```python
from build123d import *

# Parameters (mm, degrees)
SKETCH1_W           = 30.5
SKETCH1_H           = 10
BOSS_EXTRUDE1_DEPTH = 2.5
SKETCH2_W           = 35.5
SKETCH2_H           = 15
BOSS_EXTRUDE3_DEPTH = 43
SKETCH3_W           = 7
SKETCH3_H           = 3.4
CUT_EXTRUDE1_DEPTH  = 29
SKETCH4_W           = 35.5
SKETCH4_H           = 2.5
BOSS_EXTRUDE4_DEPTH = 10
SKETCH5_W           = 35.5
SKETCH5_H           = 53
SKETCH5_W_2         = 33.5
SKETCH5_H_2         = 51
BOSS_EXTRUDE5_DEPTH = 7
SKETCH6_W           = 10.5
SKETCH6_H           = 45
BOSS_EXTRUDE6_DEPTH = 7
SKETCH7_W           = 5
SKETCH7_H           = 1
SKETCH7_W_2         = 1
SKETCH7_H_2         = 2
CUT_EXTRUDE2_DEPTH  = 7
SKETCH8_W           = 1.6
SKETCH8_H           = 44
CUT_EXTRUDE3_DEPTH  = 2.5


with BuildPart() as part:
    # Sketch1 → Boss-Extrude1 (new body)
    with BuildSketch(Plane(origin=(0, 0, 0), x_dir=(1, 0, 0), z_dir=(0, 1, 0))):
        Rectangle(SKETCH1_W, SKETCH1_H)
    extrude(amount=BOSS_EXTRUDE1_DEPTH)

    # Sketch2 → Boss-Extrude3 (add)
    with BuildSketch(Plane(origin=(0, 0, 0), x_dir=(1, 0, 0), z_dir=(0, 1, 0))):
        Rectangle(SKETCH2_W, SKETCH2_H)
        Polygon((-15.25, 5), (-15.25, -5), (-10.25, -5), (-10.25, -1.6), (15.25, -1.6), (15.25, 5), align=None, mode=Mode.SUBTRACT)
    extrude(amount=BOSS_EXTRUDE3_DEPTH)

    # Sketch3 → Cut-Extrude1 (cut)
    with BuildSketch(Plane(origin=(0, 43, 0), x_dir=(1, 0, 0), z_dir=(0, 1, 0))):
        with Locations((-6.75, -3.3)):
            Rectangle(SKETCH3_W, SKETCH3_H)
    extrude(amount=-CUT_EXTRUDE1_DEPTH, mode=Mode.SUBTRACT)

    # Sketch4 → Boss-Extrude4 (add)
    with BuildSketch(Plane(origin=(0, 43, 0), x_dir=(1, 0, 0), z_dir=(0, 1, 0))):
        with Locations((0, -6.25)):
            Rectangle(SKETCH4_W, SKETCH4_H)
    extrude(amount=BOSS_EXTRUDE4_DEPTH)

    # Sketch5 → Boss-Extrude5 (add)
    with BuildSketch(Plane.XY.offset(7.5)):
        with Locations((0, 26.5)):
            Rectangle(SKETCH5_W, SKETCH5_H)
        with Locations((0, 26.5)):
            Rectangle(SKETCH5_W_2, SKETCH5_H_2, mode=Mode.SUBTRACT)
    extrude(amount=BOSS_EXTRUDE5_DEPTH)

    # Sketch6 → Boss-Extrude6 (add)
    with BuildSketch(Plane.XY.offset(7.5)):
        Polygon((-6.25, 52), (-6.25, 50), (-16.75, 50), (-16.75, 49), (-6.25, 49), (-6.25, 4), (-16.75, 4), (-16.75, 3), (-6.25, 3), (-6.25, 1), (-5.25, 1), (-5.25, 3), (5.25, 3), (5.25, 1), (6.25, 1), (6.25, 3), (16.75, 3), (16.75, 4), (6.25, 4), (6.25, 49), (16.75, 49), (16.75, 50), (6.25, 50), (6.25, 52), (5.25, 52), (5.25, 50), (-5.25, 50), (-5.25, 52), align=None)
        with Locations((0, 26.5)):
            Rectangle(SKETCH6_W, SKETCH6_H, mode=Mode.SUBTRACT)
    extrude(amount=BOSS_EXTRUDE6_DEPTH)

    # Sketch7 → Cut-Extrude2 (cut)
    with BuildSketch(Plane.XY.offset(14.5)):
        with Locations((0, 49.5)):
            Rectangle(SKETCH7_W, SKETCH7_H)
        with Locations((-11.5, 49.5)):
            Rectangle(SKETCH7_W, SKETCH7_H)
        with Locations((11.5, 49.5)):
            Rectangle(SKETCH7_W, SKETCH7_H)
        with Locations((11.5, 3.5)):
            Rectangle(SKETCH7_W, SKETCH7_H)
        with Locations((5.75, 51)):
            Rectangle(SKETCH7_W_2, SKETCH7_H_2)
        with Locations((0, 3.5)):
            Rectangle(SKETCH7_W, SKETCH7_H)
        with Locations((-11.5, 3.5)):
            Rectangle(SKETCH7_W, SKETCH7_H)
        with Locations((-5.75, 2)):
            Rectangle(SKETCH7_W_2, SKETCH7_H_2)
    extrude(amount=-CUT_EXTRUDE2_DEPTH, mode=Mode.SUBTRACT)

    # Sketch8 → Cut-Extrude3 (cut)
    with BuildSketch(Plane.XY.offset(7.5)):
        with Locations((11.5, 23)):
            Rectangle(SKETCH8_W, SKETCH8_H)
    extrude(amount=-CUT_EXTRUDE3_DEPTH, mode=Mode.SUBTRACT)


solid = part.part
```
Read the model definition and answer for the solid it produces. Units are mm, in the model's axes. A direction names the side the tool comes from. Coordinates: 2 decimals unless noted, no trailing zeros. Write each loop counter-clockwise with the first axis right and the second up, starting at its lowest first coordinate (ties: lowest second). Pieces come first, ordered by that corner, then holes. Notation, with made-up numbers: (28, 58.5) -> (38, 58.5) arc R25 cw to (38, 89.5) -> close; hole circle Ø10 at (-31.75, 66). An arc over 180 degrees is marked (long way). Answer as a JSON object with one key per item and string values.
Q1. The part is cut by section D-D on z = -2.75. Give the vertices of the cut face in (x, y), then the cut area to 3 significant figures.
The answers:
{"outline": "(-17.75, 0) -> (17.75, 0) -> (17.75, 43) -> (15.25, 43) -> (15.25, 2.5) -> (-15.25, 2.5) -> (-15.25, 43) -> (-17.75, 43) -> close", "area": "291 mm2"}
Q2. Consider line 1 (X direction, y = 27, z = 12); line 2 (Y direction, x = -16, z = 12); line 3 (X direction, y = 50.5, z = 9). Determine where each line is inside the solid, lowest interval first. Write a range as [from, to].
The answers:
{"line 1": "x = [-17.75, -16.75], [-6.25, -5.25], [5.25, 6.25], [16.75, 17.75]", "line 2": "y = [0, 1], [3, 4], [49, 50], [52, 53]", "line 3": "x = [-17.75, -16.75], [-6.25, -5.25], [16.75, 17.75]"}
Q3. The part is cut by section A-A on z = 6.5. Give the vertices of the cut face in (x, y), then the cut area to 3 significant figures.
The answers:
{"outline": "(-17.75, 0) -> (17.75, 0) -> (17.75, 53) -> (-17.75, 53) -> close; hole (10.7, 1) -> (12.3, 1) -> (12.3, 45) -> (10.7, 45) -> close", "area": "1,810 mm2"}
Q4. A tool of negligible diameter and unlimited length cuts with its end or side. For faces 5 (the flat face through (-6.25, 51, 11)), 6 (the flat face through (5, 22, 1.6)), 7 (the flat face through (17.75, 26, 3)), from which of +Z, -Z, +X, -X, +Y, -Y can it reach the whole face along a straight path? Write none if from no direction.
The answers:
{"face 5": "+Z", "face 6": "+Y", "face 7": "+Z, -Z, +X, +Y, -Y"}
Q5. Determine the mould class of faces 1 (the flat face through (11, 22, 5)), 2 (the flat face through (10.7, 23, 6)), 3 (the flat face through (0, 0, 3)), 4 (the flat face through (0, 21, -7.5)) for opening direction Y: pulls with the +Y half, pulls with the -Y half, needs draft (parallel to the pull), parting line crosses it, or undercut.
The answers:
{"face 1": "undercut", "face 2": "undercut", "face 3": "pulls with the -Y half", "face 4": "needs draft"}
Q6. The part is cut by section C-C on x = 4. Give the vertices of the cut face in (y, z), then the cut area to 3 significant figures.
The answers:
{"outline": "(0, -7.5) -> (43, -7.5) -> (43, -5) -> (2.5, -5) -> (2.5, 1.6) -> (43, 1.6) -> (43, 5) -> (53, 5) -> (53, 14.5) -> (52, 14.5) -> (52, 7.5) -> (50, 7.5) -> (50, 14.5) -> (49, 14.5) -> (49, 7.5) -> (4, 7.5) -> (4, 14.5) -> (3, 14.5) -> (3, 7.5) -> (1, 7.5) -> (1, 14.5) -> (0, 14.5) -> close", "area": "431 mm2"}
Q7. The part is cut by section B-B on y = 28.5. Give the vertices of the cut face in (x, z).
The answers:
{"outline": "(-17.75, -7.5) -> (17.75, -7.5) -> (17.75, 14.5) -> (16.75, 14.5) -> (16.75, 7.5) -> (12.3, 7.5) -> (12.3, 5) -> (10.7, 5) -> (10.7, 7.5) -> (6.25, 7.5) -> (6.25, 14.5) -> (5.25, 14.5) -> (5.25, 7.5) -> (-5.25, 7.5) -> (-5.25, 14.5) -> (-6.25, 14.5) -> (-6.25, 7.5) -> (-16.75, 7.5) -> (-16.75, 14.5) -> (-17.75, 14.5) -> close; hole (-15.25, -5) -> (15.25, -5) -> (15.25, 1.6) -> (-3.25, 1.6) -> (-3.25, 5) -> (-15.25, 5) -> close"}
Q8. A flat-ended cylindrical pin translates along its axis: pin 1 Ø1 at (x, y) = (-10.5, 38) entering from +Z. Find the tip coordinate at first contact, or state that the pin passes through.
The answers:
{"pin 1": "stops at z = 7.5"}
